```python
from build123d import *

# Parameters (mm, degrees)
SKETCH2_R                           = 1.58
BOSS_EXTRUDE1_DEPTH                 = 11.684
M3X0_5_BOTTOMING_TAPPED_HOLE1_D     = 2.5
M3X0_5_BOTTOMING_TAPPED_HOLE1_DEPTH = 3.175
M3X0_5_BOTTOMING_TAPPED_HOLE1_TIP   = 0.751075774


with BuildPart() as part:
    # Sketch1 → Revolve1 (revolve)
    with BuildSketch(Plane.XY, mode=Mode.PRIVATE) as revolve1_sk:
        Polygon((0, 0), (13.97, 0), (13.97, 19.177), (8.6995, 23.7871), (4.50215, 23.7871), (4.50215, 25.4), (0, 25.4), align=None)
    revolve(revolve1_sk.sketch.rotate(Axis((0, 0, 0), (0, 1, 0)), 90), axis=Axis((0, 0, 0), (0, 1, 0)))

    # Sketch2 → Boss-Extrude1 (add)
    with BuildSketch(Plane.XZ):
        with Locations(Location((0, 0, 0), (0, 0, 270))):
            Circle(SKETCH2_R)
    extrude(amount=BOSS_EXTRUDE1_DEPTH)

    # M3x0.5 Bottoming Tapped Hole1
    with Locations(Plane(origin=(0, 0, 0), x_dir=(-1, 0, 0), z_dir=(0, -1, 0))):
        with Locations((-8, 0), (8, 0), (0, -9.5), (0, 9.5)):
            Hole(M3X0_5_BOTTOMING_TAPPED_HOLE1_D / 2, depth=M3X0_5_BOTTOMING_TAPPED_HOLE1_DEPTH)
            with Locations((0, 0, -(M3X0_5_BOTTOMING_TAPPED_HOLE1_DEPTH + M3X0_5_BOTTOMING_TAPPED_HOLE1_TIP / 2))):  # 118° drill point
                Cone(0, M3X0_5_BOTTOMING_TAPPED_HOLE1_D / 2, M3X0_5_BOTTOMING_TAPPED_HOLE1_TIP, mode=Mode.SUBTRACT)


solid = part.part
```
Build history of the part. All positions in model axes, mm. A direction names the side the tool comes from. Give positions to 0.01 mm unless a question says otherwise; leave off trailing zeros. Order: outer loops, then holes, each group sorted by start corner. A loop starts at its lowest first (then second) coordinate and runs counter-clockwise, first axis right, second up. Notation, with made-up numbers: M 40,49.25 L 79,49.25 A33 cw 79,86.25 Z; hole C -27.5,1.25 d6. An arc over 180 degrees is marked long. Write item = value, one per line. Start each with the question number.
(1) Probe L1, parallel to X at y = 4, z = 0.5; L2, parallel to Y at x = 3.5, z = 6; L3, parallel to Z at x = -8, y = 0.8. List the from-to ranges inside material, lowest first. Write a range as [from, to].
(2) Two-plate mould, pull along X, no slides. Class faces 4 (the flat face through (0, 25.4, 0)), 5 (the conical face through (8.172, 3.796, 0.132)), 6 (the cylindrical face through (-0.16, 1.61, -10.74)), 7 (the cylindrical face through (1.567, -5.76, 0.206)): released by +X, released by -X, zero draft, split by the parting line, or undercut.
(3) Which spindle directions (+Z, -Z, +X, -X, +Y, -Y) get a long thin tool onto all of the face, cutting with end or side? Do faces 1 (the cylindrical face through (6.75, 1.61, -0.05)), 2 (the flat face through (4, 23.787, -4)), 3 (the cylindrical face through (-13.85, 9.72, 1.82)). Say none if no direction does.
(4) Slice it at A-A on y = 2. Write the cut outline in (x, z).
(5) Slice it at B-B on y = 10.5. Write the cut outline in (x, z).
(6) Slice it at C-C on y = 22. Write the cut outline in (x, z).
(7) Pin check, flat tips, straight feed: pin 1 Ø4 at (x, z) = (-8, 0) entering from -Y; pin 2 Ø4 at (x, y) = (-5, 9) entering from +Z; pin 3 Ø8 at (x, y) = (6, 7.5) entering from +Z. Stop position of each tip, or through.
Responses:
q1.L1 = [-13.96, 13.96]
q1.L2 = [0, 23.79]
q1.L3 = [-11.45, -1.25], [1.25, 11.45]
q2.face_4 = zero draft
q2.face_5 = undercut
q2.face_6 = undercut
q2.face_7 = split by the parting line
q3.face_1 = -Y
q3.face_2 = +Y
q3.face_3 = +Y, -Y
q4.outline = C 0,0 d27.94; hole C -8,0 d2.5; hole C 0,-9.5 d2.5; hole C 0,9.5 d2.5; hole C 8,0 d2.5
q5.outline = C 0,0 d27.94
q6.outline = C 0,0 d21.49
q7.pin_1 = 0
q7.pin_2 = 13.64
q7.pin_3 = 13.83
